Check sheet for the drawn part. Datum: minimum x, y, z corner. Units: mm. A direction names the side the tool comes from. Give positions to 0.01 mm unless a question says otherwise; leave off trailing zeros. Write each loop counter-clockwise with the first axis right and the second up, starting at its lowest first coordinate (ties: lowest second). Pieces come first, ordered by that corner, then holes. Notation, with made-up numbers: M 87,18 L 121,18 A19 ccw 121,50 Z; hole C 79.5,24 d6. An arc over 180 degrees is marked long. Use CSV: the item, a comma, the result in double quotes. Start each with the question number.
1. Mould release check, pull along Y, two halves, no side actions. Record for the marked faces 1 and 2: +Y half, -Y half, draft (parallel to the pull), parting line (faces both ways), or undercut.
2. Access from +Z, -Z, +X, -X, +Y, -Y to the whole of each face (thin tool, end or side, straight path). Record for the marked faces 3, 4 and 5.
3. Scan lines: line 1 (Y direction, x = 13, z = 2.1) (3 decimals); line 2 (X direction, y = 16, z = 7.5); line 3 (X direction, y = 13.75, z = 6.5). Record each from-to range of solid material in increasing order.
4. Depth check by flat-ended pin: P1, Ø2, axis at x = 5.5, y = 11, coming from the +Z side; P2, Ø4, axis at y = 3, z = 6, coming from the +X side; P3, Ø3, axis at y = 11, z = 1, coming from the -X side. Enter the tip coordinate at first touch or a pass-through.
5. Cross-section at D-D, the plane z = 3.75. Enter the section's corners in (x, y).
6. Cross-section at C-C, the plane z = 5.5. Enter the section's corners in (x, y) (3 decimals).
7. Cross-section at A-A, the plane y = 13. Enter the section's corners in (x, z) (3 decimals).
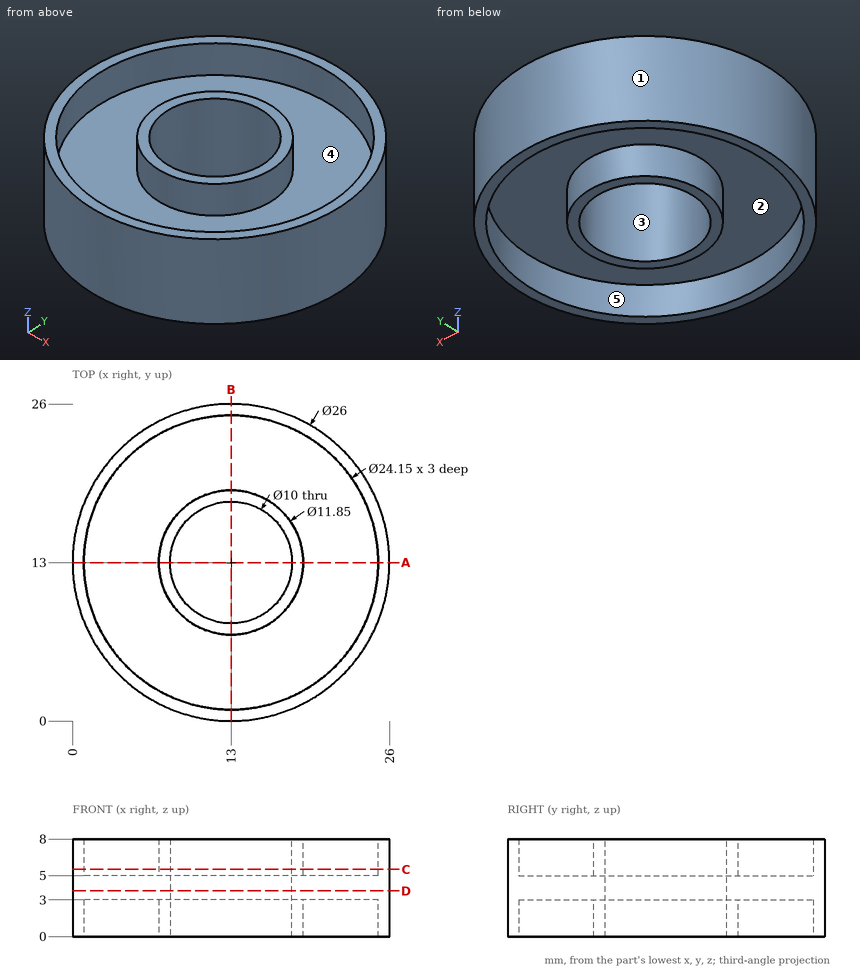
Worked answers:
1,face 1,"parting line"
1,face 2,"undercut"
2,face 3,"+Z, -Z"
2,face 4,"+Z"
2,face 5,"-Z"
3,line 1,"y = 0 to 0.925, 7.075 to 8, 18 to 18.925, 25.075 to 26"
3,line 2,"x = 0.35 to 1.3, 7.89 to 9, 17 to 18.11, 24.7 to 25.65"
3,line 3,"x = 0.02 to 0.95, 7.12 to 8.06, 17.94 to 18.88, 25.05 to 25.98"
4,P1,"stops at z = 5"
4,P2,"stops at x = 23.25"
4,P3,"stops at x = 0.01"
5,outline,"C 13,13 d26; hole C 13,13 d10"
6,outline,"C 13,13 d26; C 13,13 d11.85; hole C 13,13 d24.15; hole C 13,13 d10"
7,outline,"M 0,0 L 0.925,0 L 0.925,3 L 7.075,3 L 7.075,0 L 8,0 L 8,8 L 7.075,8 L 7.075,5 L 0.925,5 L 0.925,8 L 0,8 Z; M 18,0 L 18.925,0 L 18.925,3 L 25.075,3 L 25.075,0 L 26,0 L 26,8 L 25.075,8 L 25.075,5 L 18.925,5 L 18.925,8 L 18,8 Z"
